Input: part model. Units: mm. Frame: model coordinates. A direction names the side the tool comes from. Coordinates: 2 decimals unless noted, no trailing zeros. Order: outer loops, then holes, each group sorted by start corner. A loop starts at its lowest first (then second) coordinate and runs counter-clockwise, first axis right, second up. Notation, with made-up numbers: M 56,88.25 L 90,88.25 A24 ccw 90,109.25 Z; hole C 89,77 d7. An arc over 180 degrees is marked long. Answer in a Markdown table with one row per item.
from build123d import *

# Parameters (mm, degrees)
PAD_DEPTH            = 40
SKETCH001_R          = 10
PAD001_DEPTH         = 20
SKETCH002_R          = 2
POCKET_DEPTH         = 32.001
SKETCH003_R          = 2
POCKET001_DEPTH      = 15.001
POCKET001_DEPTH_BACK = -15.001
GROOVE_ANGLE         = -180


with BuildPart() as part:
    # Sketch → Pad (new body)
    with BuildSketch(Plane.XY):
        with BuildLine():
            ThreePointArc((0, 10), (-10, 0), (0, -10))
            Line((0, -10), (0, -15))
            Line((-27, -15), (0, -15))
            ThreePointArc((-32, -10), (-30.535534, -13.535534), (-27, -15))
            Line((-32, 10), (-32, -10))
            ThreePointArc((-27, 15), (-30.535534, 13.535534), (-32, 10))
            Line((-27, 15), (0, 15))
            Line((0, 15), (0, 10))
        make_face()
    extrude(amount=PAD_DEPTH)

    # Sketch001 → Pad001 (join)
    with BuildSketch(Plane.XY.offset(40)):
        with Locations((-20, 0)):
            Circle(SKETCH001_R)
    extrude(amount=PAD001_DEPTH)

    # Sketch002 → Pocket (cut, through all)
    with BuildSketch(Plane.YZ):
        with Locations((-15, 20)):
            Circle(SKETCH002_R)
        with Locations((15, 20)):
            Circle(SKETCH002_R)
        with Locations((-15, 30)):
            Circle(SKETCH002_R)
        with Locations((-15, 10)):
            Circle(SKETCH002_R)
        with Locations((15, 30)):
            Circle(SKETCH002_R)
        with Locations((15, 10)):
            Circle(SKETCH002_R)
    extrude(amount=-POCKET_DEPTH, mode=Mode.SUBTRACT)

    # Sketch003 → Pocket001 (cut, two sides)
    with BuildSketch(Plane.XZ) as pocket001_sk:
        with Locations((-32, 20)):
            Circle(SKETCH003_R)
        with Locations((-32, 30)):
            Circle(SKETCH003_R)
        with Locations((-32, 10)):
            Circle(SKETCH003_R)
    extrude(amount=-POCKET001_DEPTH, mode=Mode.SUBTRACT)
    extrude(pocket001_sk.sketch, amount=-POCKET001_DEPTH_BACK, mode=Mode.SUBTRACT)

    # Sketch004 → Groove (revolve, cut)
    with BuildSketch(Plane.YZ.offset(-20)):
        with BuildLine():
            ThreePointArc((-15, 8), (-13, 10), (-15, 12))
            Line((-15, 12), (-25, 12))
            Line((-25, 12), (-25, 8))
            Line((-25, 8), (-15, 8))
        make_face()
        with BuildLine():
            ThreePointArc((-15, 28), (-13, 30), (-15, 32))
            Line((-25, 32), (-15, 32))
            Line((-25, 32), (-25, 28))
            Line((-25, 28), (-15, 28))
        make_face()
        with BuildLine():
            ThreePointArc((-15, 18), (-13, 20), (-15, 22))
            Line((-15, 22), (-25, 22))
            Line((-25, 22), (-25, 18))
            Line((-25, 18), (-15, 18))
        make_face()
    revolve(axis=Axis((-20, 0, 0), (0, 0, 1)), revolution_arc=GROOVE_ANGLE, mode=Mode.SUBTRACT)


solid = part.part
1) Cut plane B-B, the plane y = -5. Output: boundary loops of the cut face in (x, z).
Resolved:
| item | result |
|---|---|
| outline | M -32,0 L -8.66,0 L -8.66,40 L -11.34,40 L -11.34,60 L -28.66,60 L -28.66,40 L -32,40 L -32,32 A2 cw -32,28 L -32,22 A2 cw -32,18 L -32,12 A2 cw -32,8 Z |
2) Cut plane D-D, the plane z = 45. Output: boundary loops of the cut face in (x, y), and give its area (3 significant figures).
Resolved:
| item | result |
|---|---|
| outline | C -20,0 d20 |
| area | 314 mm2 |
3) Cut plane A-A, the plane z = 4.5. Output: boundary loops of the cut face in (x, y), and give its area (3 significant figures).
Resolved:
| item | result |
|---|---|
| outline | M -32,-10 A5 ccw -27,-15 L 0,-15 L 0,-10 A10 cw 0,10 L 0,15 L -27,15 A5 ccw -32,10 Z |
| area | 792 mm2 |
4) Mould query, pull axis Z, two halves, no side actions, for faces 4 (the face through (-12, 7, 40)), 5 (the face through (-29, -13, 28)), 6 (the face through (-30, 14, 36)). Classes: +Z half, -Z half, draft (parallel to the pull), parting line (faces both ways), or undercut.
Resolved:
| item | result |
|---|---|
| face 4 | +Z half |
| face 5 | undercut |
| face 6 | draft |
5) Reachability of faces 1 (the face through (-10.46, 3, 49.86)), 2 (the face through (-28, 13, 18)), 3 (the face through (-10, 0, 20)) from +Z, -Z, +X, -X, +Y, -Y: full face, straight path, thin tool, end or side. Return the list, or none.
Resolved:
| item | result |
|---|---|
| face 1 | +Z |
| face 2 | -X, +Y |
| face 3 | +Z, -Z, +X |
6) Material intervals for probe 1 along Z at (x, y) = (-23, -12); probe 2 along Y at (x, z) = (-5, 13); probe 3 along Y at (x, z) = (-2.5, 18.5), sorted ascending.
Resolved:
| item | result |
|---|---|
| probe 1 | z = 0 to 40 |
| probe 2 | y = -15 to -8.66, 8.66 to 15 |
| probe 3 | y = -13.68 to -9.68, 9.68 to 13.68 |
7) Contact query for flat-ended pins moving along their axis: pin 1 (1 mm diameter, centred on x = -13.5, z = 41.5, fed in from +Y); pin 2 (5 mm diameter, centred on x = -26, y = -10.5, fed in from +Z); pin 3 (3 mm diameter, centred on x = -28, y = 12.5, fed in from +Z); pin 4 (10 mm diameter, centred on x = -23.5, z = 50.5, fed in from +Y). Output: stop coordinate, or through.
Resolved:
| item | result |
|---|---|
| pin 1 | stops at y = 8 |
| pin 2 | stops at z = 60 |
| pin 3 | stops at z = 40 |
| pin 4 | stops at y = 10 |
8) Cut plane C-C, the plane x = -18. Output: boundary loops of the cut face in (y, z).
Resolved:
| item | result |
|---|---|
| outline | M -15,0 L 15,0 L 15,8 A2 cw 15,12 L 15,18 A2 cw 15,22 L 15,28 A2 cw 15,32 L 15,40 L 9.8,40 L 9.8,60 L -9.8,60 L -9.8,40 L -15,40 L -15,32 A2 cw -15,28 L -15,22 A2 cw -15,18 L -15,12 A2 cw -15,8 Z |
